from build123d import *

# Parameters (mm, degrees)
CROQUIS1_W              = 1000
CROQUIS1_H              = 400
SALIENTE_EXTRUIR1_DEPTH = 400
CROQUIS2_R              = 140
CORTAR_EXTRUIR1_DEPTH   = 1000
CROQUIS3_W              = 500
CROQUIS3_H              = 200
CORTAR_EXTRUIR2_DEPTH   = 400
CROQUIS4_R              = 50
SALIENTE_EXTRUIR2_DEPTH = 400
SALIENTE_EXTRUIR2_TAPER = 4


with BuildPart() as part:
    # Croquis1 → Saliente-Extruir1 (new body)
    with BuildSketch(Plane.XY):
        with Locations((500, 200)):
            Rectangle(CROQUIS1_W, CROQUIS1_H)
    extrude(amount=SALIENTE_EXTRUIR1_DEPTH)

    # Croquis2 → Cortar-Extruir1 (cut)
    with BuildSketch(Plane(origin=(1000, 0, 0), x_dir=(0, 0, -1), z_dir=(1, 0, 0))):
        with Locations((-200, 200)):
            Circle(CROQUIS2_R)
    extrude(amount=-CORTAR_EXTRUIR1_DEPTH, mode=Mode.SUBTRACT)

    # Croquis3 → Cortar-Extruir2 (cut)
    with BuildSketch(Plane.XZ):
        with Locations((500, 200)):
            Rectangle(CROQUIS3_W, CROQUIS3_H)
    extrude(amount=-CORTAR_EXTRUIR2_DEPTH, mode=Mode.SUBTRACT)

    # Croquis4 → Saliente-Extruir2 (add)
    with BuildSketch(Plane.XZ):
        with Locations((875, 200)):
            Circle(CROQUIS4_R)
    extrude(amount=SALIENTE_EXTRUIR2_DEPTH, taper=SALIENTE_EXTRUIR2_TAPER)


solid = part.part
The listing builds one solid part. Answer for the finished solid, in the listing's coordinates (mm). A direction names the side the tool comes from. Give positions to 0.01 mm unless a question says otherwise; leave off trailing zeros. Order: outer loops, then holes, each group sorted by start corner. A loop starts at its lowest first (then second) coordinate and runs counter-clockwise, first axis right, second up. Notation, with made-up numbers: (30.5, -18.5) -> (52.5, -18.5) arc R38 ccw to (52.5, 19.5) -> close; hole circle Ø8 at (89, 6.25). An arc over 180 degrees is marked (long way). Put each result on its own line as item: value.
Item 1: Given P1, Ø12, axis at x = 829, z = 163, coming from the -Y side, flat-ended and moving along its own axis, determine where the tip first touches the part or whether it passes through.
Established:
P1: stops at y = 0
Item 2: A cutting plane is placed at A-A on x = 592. Give the vertices of the cut face in (y, z).
Established:
outline: (0, 0) -> (400, 0) -> (400, 100) -> (297.98, 100) arc R140 cw to (102.02, 100) -> (0, 100) -> close; (0, 300) -> (102.02, 300) arc R140 cw to (297.98, 300) -> (400, 300) -> (400, 400) -> (0, 400) -> close
Item 3: Straight lines are drawn through the part: line 1 (X direction, y = 27, z = 126.5); line 2 (Y direction, x = 770.5, z = 200); line 3 (Y direction, x = 205.5, z = 366.5). For each, find the intervals that lie inside material, in ascending order.
Established:
line 1: x = 0 to 250, 750 to 1000
line 2: y = 0 to 60, 340 to 400
line 3: y = 0 to 400
Item 4: A cutting plane is placed at C-C on x = 214.5. Give the vertices of the cut face in (y, z).
Established:
outline: (0, 0) -> (400, 0) -> (400, 400) -> (0, 400) -> close; hole circle Ø280 at (200, 200)
Item 5: For faces 4 (the face through (250, 360, 199)), 5 (the face through (493, 203, 0)), determine the directions among +Z, -Z, +X, -X, +Y, -Y from which every point of the face is accessible in a straight line to the end or side of a thin tool.
Established:
face 4: +Y, -Y
face 5: -Z, +X, -X, +Y, -Y
Item 6: A cutting plane is placed at B-B on y = 200. Give the vertices of the cut face in (x, z).
Established:
outline: (0, 0) -> (1000, 0) -> (1000, 60) -> (0, 60) -> close; (0, 340) -> (1000, 340) -> (1000, 400) -> (0, 400) -> close
Item 7: For a pull along Z with two mould halves and no side action, classify faces 1 (the face through (875, -400, 200)), 2 (the face through (909.165, -202.8, 210.759)), 3 (the face through (507, 206.156, 339.865)) as released by +Z, released by -Z, zero draft, split by the parting line, or undercut.
Established:
face 1: zero draft
face 2: split by the parting line
face 3: undercut
Item 8: A cutting plane is placed at D-D on z = 200. Count the separate pieces of the cut face and the enclosed holes in it, plus the area to 3 significant figures.
Established:
separate pieces: 4
enclosed holes: 0
area: 88,800 mm^2
